Check sheet for the modelled part. Datum: model origin and axes. Units: mm. Face numbers are marked on the shaded views. A direction names the side the tool comes from. Give positions to 0.01 mm unless a question says otherwise; leave off trailing zeros. Write each loop counter-clockwise with the first axis right and the second up, starting at its lowest first coordinate (ties: lowest second). Pieces come first, ordered by that corner, then holes. Notation, with made-up numbers: (81, 86.25) -> (131, 86.25) arc R15 cw to (131, 92.25) -> close; hole circle Ø7 at (69.5, 75.5). An arc over 180 degrees is marked (long way). Use a Markdown table: item, result. Add a question column.
1. Cross-section at A-A (z = 6). Enter the section's corners in (x, y) (3 decimals).
2. Gauge pin test, flat ends, axial feed: P1, Ø2.5, axis at x = 53.5, z = 6, coming from the +Y side; P2, Ø2.5, axis at y = -12.5, z = 45.5, coming from the -X side; P3, Ø5, axis at x = 5, z = 47, coming from the -Y side; P4, Ø4, axis at x = 24.5, z = 14, coming from the +Y side. Record the tip position at first contact, or that the pin passes through.
3. Scan lines: probe 1 along Z at (x, y) = (5, -2.75) (3 decimals); probe 2 along X at (y, z) = (-4.75, 28); probe 3 along X at (y, z) = (0, 39). Record each from-to range of solid material in increasing order. Write a range as [from, to].
4. Cross-section at C-C (x = 5). Enter the section's corners in (y, z) (3 decimals).
5. Cross-section at B-B (y = -6). Enter the section's corners in (x, z) (3 decimals), then the cut area to 3 significant figures.
6. Set-up check for the marked faces 1 and 2: record each of +Z, -Z, +X, -X, +Y, -Y from which the full face is reachable in a straight line by a thin tool's end or side.
7. Cross-section at D-D (z = 47). Enter the section's corners in (x, y) (3 decimals), then the cut area to 3 significant figures.
from build123d import *

# Parameters (mm, degrees)
SKETCH1_W                                  = 58.5
SKETCH1_H                                  = 20
BOSS_EXTRUDE1_DEPTH                        = 53
CUT_EXTRUDE2_DEPTH                         = 24.7
CUT_EXTRUDE3_DEPTH                         = 32.4
SKETCH8_W                                  = 10
SKETCH8_H                                  = 8
CUT_EXTRUDE6_DEPTH                         = 3
SKETCH7_R                                  = 1.585
CUT_EXTRUDE5_DEPTH                         = 92.5
MIRROR1_AT_THE_SECOND_PLANE_COPY_1_SKETC_W = 10
MIRROR1_AT_THE_SECOND_PLANE_COPY_1_SKETC_H = 8
MIRROR1_AT_THE_SECOND_PLANE_COPY_1_DEPTH   = 3


with BuildPart() as part:
    # Sketch1 → Boss-Extrude1 (new body)
    with BuildSketch(Plane.XY):
        with Locations((29.25, -3.609195402)):
            Rectangle(SKETCH1_W, SKETCH1_H)
    extrude(amount=BOSS_EXTRUDE1_DEPTH)

    # Sketch3 → Cut-Extrude2 (cut)
    with BuildSketch(Plane.XY.offset(53)):
        with BuildLine():
            Line((14.434183752, 6.390804598), (44.05, 6.390804598))
            ThreePointArc((44.05, 6.390804598), (29.242091876, -8.417103526), (14.434183752, 6.390804598))
        make_face()
    extrude(amount=-CUT_EXTRUDE2_DEPTH, mode=Mode.SUBTRACT)

    # Sketch5 → Cut-Extrude3 (cut)
    with BuildSketch(Plane(origin=(0, 0, 0), x_dir=(-1, 0, 0), z_dir=(0, 0, -1))):
        with BuildLine():
            Line((-43.05, 6.390804598), (-15.45, 6.390804598))
            ThreePointArc((-15.45, 6.390804598), (-29.25, -7.409195402), (-43.05, 6.390804598))
        make_face()
    extrude(amount=-CUT_EXTRUDE3_DEPTH, mode=Mode.SUBTRACT)

    # Sketch8 → Cut-Extrude6 (cut)
    with BuildSketch(Plane(origin=(0, -13.609195402, 0), x_dir=(-1, 0, 0), z_dir=(0, -1, 0))):
        with Locations((-53.5, -6)):
            Rectangle(SKETCH8_W, SKETCH8_H)
    cut_extrude6 = extrude(amount=-CUT_EXTRUDE6_DEPTH, mode=Mode.SUBTRACT)

    # Sketch7 → Cut-Extrude5 (cut)
    with BuildSketch(Plane(origin=(0, -13.609195402, 0), x_dir=(-1, 0, 0), z_dir=(0, -1, 0))):
        with Locations(Location((-53.5, -47, 0), (0, 0, 180))):
            Circle(SKETCH7_R)
        with Locations(Location((-53.5, -6, 0), (0, 0, 180))):
            Circle(SKETCH7_R)
        with Locations(Location((-5, -6, 0), (0, 0, 180))):
            Circle(SKETCH7_R)
        with Locations(Location((-5, -47, 0), (0, 0, 180))):
            Circle(SKETCH7_R)
    extrude(amount=-CUT_EXTRUDE5_DEPTH, mode=Mode.SUBTRACT)

    # Mirror1: Cut-Extrude6 across plane
    add(cut_extrude6.mirror(Plane.XY.offset(26.5)), mode=Mode.SUBTRACT)

    # Mirror1 at the second plane: Cut-Extrude6 across plane
    add(cut_extrude6.mirror(Plane.ZY.offset(-29.25)), mode=Mode.SUBTRACT)

    # Mirror1 at the second plane copy 1 sketc → Mirror1 at the second plane copy 1 (cut)
    with BuildSketch(Plane(origin=(58.5, -13.609195402, 53), x_dir=(1, 0, 0), z_dir=(0, -1, 0))):
        with Locations((-53.5, -6)):
            Rectangle(MIRROR1_AT_THE_SECOND_PLANE_COPY_1_SKETC_W, MIRROR1_AT_THE_SECOND_PLANE_COPY_1_SKETC_H)
    extrude(amount=-MIRROR1_AT_THE_SECOND_PLANE_COPY_1_DEPTH, mode=Mode.SUBTRACT)


solid = part.part
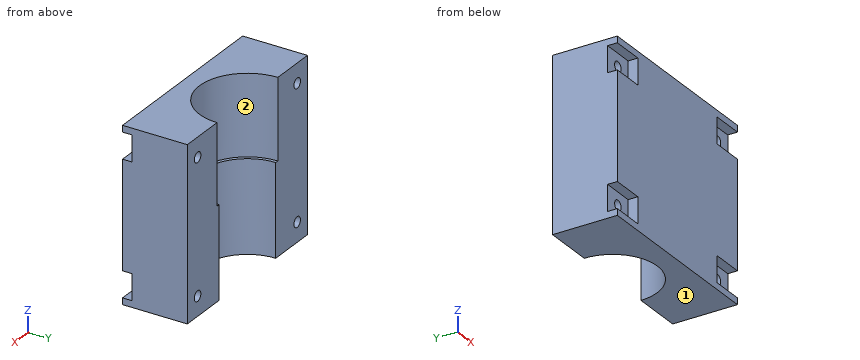
Worked answers:
| question | item | result |
|---|---|---|
| 1 | outline | (0, -10.609) -> (3.415, -10.609) -> (3.415, 6.391) -> (0, 6.391) -> close; (6.585, -10.609) -> (10, -10.609) -> (10, -13.609) -> (48.5, -13.609) -> (48.5, -10.609) -> (51.915, -10.609) -> (51.915, 6.391) -> (43.05, 6.391) arc R13.8 cw to (15.45, 6.391) -> (6.585, 6.391) -> close; (55.085, -10.609) -> (58.5, -10.609) -> (58.5, 6.391) -> (55.085, 6.391) -> close |
| 2 | P1 | passes through |
| 2 | P2 | stops at x = 10 |
| 2 | P3 | stops at y = -10.61 |
| 2 | P4 | stops at y = -5.65 |
| 3 | probe 1 | z = [0, 4.415], [7.585, 45.415], [48.585, 53] |
| 3 | probe 2 | x = [0, 21.11], [37.39, 58.5] |
| 3 | probe 3 | x = [0, 15.88], [42.6, 58.5] |
| 4 | outline | (-13.609, 0) -> (6.391, 0) -> (6.391, 4.415) -> (-10.609, 4.415) -> (-10.609, 2) -> (-13.609, 2) -> close; (-13.609, 10) -> (-10.609, 10) -> (-10.609, 7.585) -> (6.391, 7.585) -> (6.391, 45.415) -> (-10.609, 45.415) -> (-10.609, 43) -> (-13.609, 43) -> close; (-13.609, 51) -> (-10.609, 51) -> (-10.609, 48.585) -> (6.391, 48.585) -> (6.391, 53) -> (-13.609, 53) -> close |
| 5 | outline | (0, 0) -> (23.175, 0) -> (23.175, 28.3) -> (21.134, 28.3) -> (21.134, 53) -> (0, 53) -> close; (35.325, 0) -> (58.5, 0) -> (58.5, 53) -> (37.35, 53) -> (37.35, 28.3) -> (35.325, 28.3) -> close; hole circle Ø3.17 at (5, 6); hole circle Ø3.17 at (5, 47); hole circle Ø3.17 at (53.5, 6); hole circle Ø3.17 at (53.5, 47) |
| 5 | area | 2,320 mm² |
| 6 | face 1 | -Z, +X, -X, +Y, -Y |
| 6 | face 2 | +Z, +Y |
| 7 | outline | (0, -10.609) -> (3.415, -10.609) -> (3.415, 6.391) -> (0, 6.391) -> close; (6.585, -10.609) -> (10, -10.609) -> (10, -13.609) -> (48.5, -13.609) -> (48.5, -10.609) -> (51.915, -10.609) -> (51.915, 6.391) -> (44.05, 6.391) arc R14.808 cw to (14.434, 6.391) -> (6.585, 6.391) -> close; (55.085, -10.609) -> (58.5, -10.609) -> (58.5, 6.391) -> (55.085, 6.391) -> close |
| 7 | area | 658 mm² |
